from build123d import *

# Parameters (mm, degrees)
SKETCH1_W           = 120
SKETCH1_H           = 120
BOSS_EXTRUDE1_DEPTH = 90
FILLET1_R           = 10
SHELL1_T            = -4
BOSS_EXTRUDE3_START = 20
BOSS_EXTRUDE3_DEPTH = 20


with BuildPart() as part:
    # Sketch1 → Boss-Extrude1 (new body)
    with BuildSketch(Plane.XY):
        with Locations((60, 60)):
            Rectangle(SKETCH1_W, SKETCH1_H)
    extrude(amount=BOSS_EXTRUDE1_DEPTH)

    # Fillet1
    fillet1_edges = [part.edges().sort_by_distance(p)[0] for p in [
        (0, 0, 45),
        (120, 0, 45),
        (120, 120, 45),
        (0, 120, 45),
    ]]
    fillet(fillet1_edges, radius=FILLET1_R)

    # Shell1
    shell1_openings = [part.faces().sort_by_distance(p)[0] for p in [
        (60, 60, 90),
    ]]
    offset(amount=SHELL1_T, openings=shell1_openings, kind=Kind.INTERSECTION)

    # Sketch2 → Boss-Extrude3 (add)
    with BuildSketch(Plane.XY.offset(90).offset(BOSS_EXTRUDE3_START)):
        with BuildLine():
            ThreePointArc((10, 118), (4.343145751, 115.656854249), (2, 110))
            Line((2, 110), (2, 10))
            ThreePointArc((2, 10), (4.343145751, 4.343145751), (10, 2))
            Line((10, 2), (110, 2))
            ThreePointArc((110, 2), (115.656854249, 4.343145751), (118, 10))
            Line((118, 10), (118, 110))
            ThreePointArc((118, 110), (115.656854249, 115.656854249), (110, 118))
            Line((110, 118), (10, 118))
        make_face()
        with BuildLine():
            ThreePointArc((116, 10), (114.242640687, 5.757359313), (110, 4))
            Line((110, 4), (10, 4))
            ThreePointArc((10, 4), (5.757359313, 5.757359313), (4, 10))
            Line((4, 10), (4, 110))
            ThreePointArc((4, 110), (5.757359313, 114.242640687), (10, 116))
            Line((10, 116), (110, 116))
            ThreePointArc((110, 116), (114.242640687, 114.242640687), (116, 110))
            Line((116, 110), (116, 10))
        make_face(mode=Mode.SUBTRACT)
    extrude(amount=-BOSS_EXTRUDE3_DEPTH)


solid = part.part
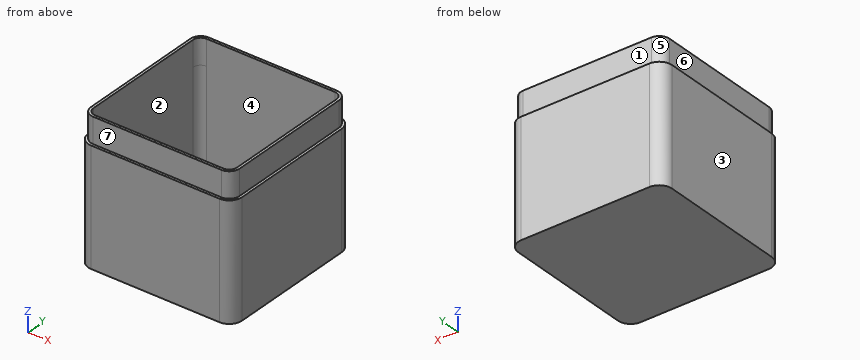
The model under review builds one solid part; all positions refer to its coordinate system, in mm. Face numbers are marked on the shaded views. A direction names the side the tool comes from. Give positions to 0.01 mm unless a question says otherwise; leave off trailing zeros. Order: outer loops, then holes, each group sorted by start corner. A loop starts at its lowest first (then second) coordinate and runs counter-clockwise, first axis right, second up. Notation, with made-up numbers: M -22,48 L -13,48 A9 ccw -13,59 Z; hole C 69,-19 d8. An arc over 180 degrees is marked long. Answer in a Markdown table with one row per item. Add a question column.
1. To check wall thickness, follow line 1 along X through (y, z) = (68.5, 37.5); line 2 along X through (y, z) = (44, 102). State the ranges of each line that lie inside material, in increasing order.
2. Add section A-A on z = 71.5. State the section outline as (x, y) points, plus the area to 3 significant figures.
3. Machinability: for the marked faces 4, 5, 6 and 7, which of the approach directions +Z, -Z, +X, -X, +Y, -Y give a long, thin tool a straight path to every point of the face, cutting with its end or side? Answer none if there is none.
4. For pin 1 Ø12 at (x, y) = (36.5, 41.5) entering from +Z; pin 2 Ø6 at (x, z) = (39, 102) entering from +Y; pin 3 Ø16 at (y, z) = (63, 102.5) entering from +X, all flat-tipped, find the tip position at first contact; note any pin that passes through.
5. Add section D-D on z = 95. State the section outline as (x, y) points.
6. Add section B-B on y = 84.5. State the section outline as (x, z) points.
7. Mouldability with a two-part tool opening along Y and no side actions: class the marked faces 1, 2 and 3 as released by +Y, released by -Y, zero draft, split by the parting line, or undercut.
The answers:
| question | item | result |
|---|---|---|
| 1 | line 1 | 0 to 4, 116 to 120 |
| 1 | line 2 | 2 to 4, 116 to 118 |
| 2 | outline | M 0,10 A10 ccw 10,0 L 110,0 A10 ccw 120,10 L 120,110 A10 ccw 110,120 L 10,120 A10 ccw 0,110 Z; hole M 4,10 A6 ccw 10,4 L 110,4 A6 ccw 116,10 L 116,110 A6 ccw 110,116 L 10,116 A6 ccw 4,110 Z |
| 2 | area | 1,800 mm2 |
| 3 | face 4 | +Z |
| 3 | face 5 | +Z, -X, +Y |
| 3 | face 6 | +Z, -X, +Y, -Y |
| 3 | face 7 | +Z, +X, -X, -Y |
| 4 | pin 1 | z = 4 |
| 4 | pin 2 | y = 118 |
| 4 | pin 3 | x = 118 |
| 5 | outline | M 2,10 A8 ccw 10,2 L 110,2 A8 ccw 118,10 L 118,110 A8 ccw 110,118 L 10,118 A8 ccw 2,110 Z; hole M 4,10 A6 ccw 10,4 L 110,4 A6 ccw 116,10 L 116,110 A6 ccw 110,116 L 10,116 A6 ccw 4,110 Z |
| 6 | outline | M 0,0 L 120,0 L 120,90 L 118,90 L 118,110 L 116,110 L 116,4 L 4,4 L 4,110 L 2,110 L 2,90 L 0,90 Z |
| 7 | face 1 | released by +Y |
| 7 | face 2 | undercut |
| 7 | face 3 | zero draft |
